Input: part model. Units: mm. Frame: model coordinates. Round coordinates to 2 decimals unless told otherwise and drop trailing zeros. Loops run counter-clockwise (first coordinate to the right, second up) from the corner with the lowest first, then second, coordinate; pieces in that order, holes last.
1) Section B-B, the plane y = 9. Return loops of the section in (x, z), and give its area (3 significant figures).
2) Section A-A, the plane z = 38.05. Return loops of the section in (x, y), and give its area (3 significant figures).
3) Ray query, line 1 along Z through (x, y) = (0.6, 9.75); line 2 along Z through (x, y) = (2.85, 9.5); line 3 along Y through (x, z) = (1.35, 38.05). Return the intervals inside material, ascending.
4) Section D-D, the plane z = 8.05. Return loops of the section in (x, y), and give its area (3 significant figures).
5) First-contact query: pin 1 (2 mm diameter, centred on x = 1.5, y = 14.5, fed in from +Z); pin 2 (2 mm diameter, centred on x = 2, y = 9.5, fed in from -Z); pin 3 (2.5 mm diameter, centred on y = 9, z = 38.05, fed in from +X); pin 4 (1.5 mm diameter, centred on x = 3.5, z = 36, fed in from +Y). Flat tips, straight axial feed; report the tip coordinate or a pass-through.
6) Section C-C, the plane x = 1.45. Return loops of the section in (y, z), and give its area (3 significant figures).
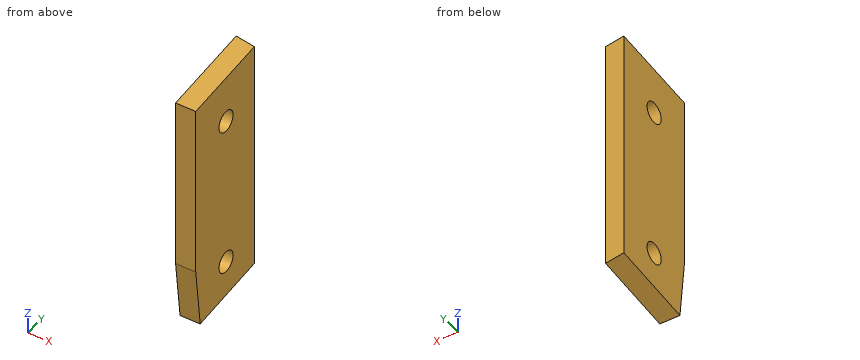
from build123d import *

# Parameters (mm, degrees)
EXTRUSION1_DEPTH  = 48.3
TROU_TARAUD_M51_D = 4.2
EXTRUSION2_DEPTH  = 52.7
EXTRUSION3_DEPTH  = 52.7


with BuildPart() as part:
    # Esquisse1 → Extrusion1 (new body)
    with BuildSketch(Plane.XY):
        Polygon((0, 0), (4, 0), (4, 17.437836661), (0, 18), align=None)
    extrude(amount=EXTRUSION1_DEPTH)

    # Trou taraudé M51 (through all)
    with Locations(Plane(origin=(4, 0, 0), x_dir=(0, 0, -1), z_dir=(1, 0, 0))):
        with Locations((-8.05, 9), (-38.05, 9)):
            Hole(TROU_TARAUD_M51_D / 2)

    # Esquisse4 → Extrusion2 (cut, through all)
    with BuildSketch(Plane.ZY):
        Polygon((48.3, 18), (46.312781499, 0), (48.3, 0), align=None)
        Polygon((0, 0), (0, 1.324812334), (12, 0), align=None)
    extrude(amount=-EXTRUSION2_DEPTH, mode=Mode.SUBTRACT)

    # Esquisse5 → Extrusion3 (cut, through all)
    with BuildSketch(Plane.ZY):
        Polygon((0, 1.324812334), (2, 18), (0, 18), align=None)
    extrude(amount=-EXTRUSION3_DEPTH, mode=Mode.SUBTRACT)


solid = part.part
Final values:
1. outline: (0, 0.92) - (4, 0.92) - (4, 5.95) - (0, 5.95) - close; (0, 10.15) - (4, 10.15) - (4, 35.95) - (0, 35.95) - close; (0, 40.15) - (4, 40.15) - (4, 47.31) - (0, 47.31) - close
1. area: 152 mm2
2. outline: (0, 0) - (4, 0) - (4, 6.9) - (0, 6.9) - close; (0, 11.1) - (4, 11.1) - (4, 17.44) - (0, 18) - close
2. area: 54.1 mm2
3. line 1: z = 1.01 to 6.09, 10.01 to 36.09, 40.01 to 47.39
3. line 2: z = 0.98 to 6.01, 10.09 to 36.01, 40.09 to 47.36
3. line 3: y = 0 to 6.9, 11.1 to 17.81
4. outline: (0, 0.44) - (4, 0.44) - (4, 6.9) - (0, 6.9) - close; (0, 11.1) - (4, 11.1) - (4, 17.44) - (0, 18) - close
4. area: 52.3 mm2
5. pin 1: stops at z = 48.02
5. pin 2: stops at z = 0.86
5. pin 3: passes through
5. pin 4: stops at y = 17.61
6. outline: (0, 12) - (1.32, 0) - (17.8, 1.98) - (17.8, 48.28) - (0, 46.31) - close; hole circle Ø4.2 at (9, 8.05); hole circle Ø4.2 at (9, 38.05)
6. area: 790 mm2
